Part model, mm, in its own coordinate system. A direction names the side the tool comes from. Give positions to 0.01 mm unless a question says otherwise; leave off trailing zeros. Write each loop counter-clockwise with the first axis right and the second up, starting at its lowest first coordinate (ties: lowest second). Pieces come first, ordered by that corner, then holes. Notation, with made-up numbers: (73.5, 71) - (130.5, 71) arc R24 ccw to (130.5, 93) - close; hole circle Ø5 at (18, 8). An arc over 180 degrees is marked (long way). Answer as a JSON object with one key per item and string values. Group by question number.
```python
from build123d import *


with BuildPart() as part:
    # Sketch1 → Revolve1 (revolve)
    with BuildSketch(Plane.XY):
        with BuildLine():
            Line((-27, 10), (12, 10))
            ThreePointArc((12, 10), (12.707106781, 10.292893219), (13, 11))
            Line((13, 11), (13, 14))
            Line((13, 14), (27, 14))
            Line((27, 14), (27, 17.5))
            Line((27, 17.5), (14, 17.5))
            Line((14, 17.5), (14, 19))
            Line((14, 19), (0, 19))
            Line((0, 19), (0, 21))
            Line((0, 21), (-2, 21))
            Line((-2, 21), (-2, 20.229142798))
            ThreePointArc((-2, 20.229142798), (-2.062403045, 20.049198361), (-2.222815548, 19.946524269))
            Line((-2.222815548, 19.946524269), (-27, 14))
            Line((-27, 14), (-27, 10))
        make_face()
    revolve(axis=Axis((-27, 0, 0), (1, 0, 0)))


solid = part.part
```
1) Mould opens along Z. For faces 4 (the flat face through (13, -6.2, -9.3)), 5 (the cylindrical face through (20.098, 12.932, -5.362)), 6 (the cylindrical face through (-1.01, 20.03, 6.31)), 7 (the flat face through (27, 8, 12)) say: pulls with the +Z half, pulls with the -Z half, needs draft (parallel to the pull), parting line crosses it, or undercut.
2) Drop flat-ended pins along their axis: P1, Ø6, axis at x = -19, z = -13.5, coming from the +Y side; P2, Ø1.5, axis at x = -11, y = -7, coming from the -Z side; P3, Ø6, axis at x = -17.5, z = 4, coming from the -Y side. Give the stop position or say it passes through.
3) Probe line 1 (Z direction, x = 22.5, y = 0); line 2 (X direction, y = -4, z = 13); line 3 (X direction, y = 15.5, z = 13). List the from-to ranges inside material, lowest first.
4) Band-saw the part on C-C (x = -13). List the corners of the cut face in (y, z).
5) Band-saw the part on D-D (x = -21). List the corners of the cut face in (y, z), plus the area to 3 significant figures.
6) Which spindle directions (+Z, -Z, +X, -X, +Y, -Y) get a long thin tool onto all of the face, cutting with end or side? Do faces 1 (the flat face through (-27, -3, 10)), 2 (the flat face through (-2, -11, 17.2)), 3 (the cylindrical face through (20.409, -13.887, -10.648)). Say none if no direction does.
7) Band-saw the part on A-A (z = 0). List the corners of the cut face in (x, y), plus the area to 3 significant figures.
Verdict:
{
 "1": {"face 4": "undercut", "face 5": "undercut", "face 6": "parting line crosses it", "face 7": "needs draft"},
 "2": {"P1": "y = 12.14", "P2": "z = -16.77", "P3": "y = -16.72"},
 "3": {"line 1": "-17.5 to -14, 14 to 17.5", "line 2": "-27 to 13", "line 3": "-2 to 0"},
 "4": {"outline": "circle Ø34.72 at (0, 0); hole circle Ø20 at (0, 0)"},
 "5": {"outline": "circle Ø30.88 at (0, 0); hole circle Ø20 at (0, 0)", "area": "435 mm2"},
 "6": {"face 1": "+Z, -Z, -X, +Y, -Y", "face 2": "-X", "face 3": "+X"},
 "7": {"outline": "(-27, -14) - (-2.22, -19.95) arc R0.29 cw to (-2, -20.23) - (-2, -21) - (0, -21) - (0, -19) - (14, -19) - (14, -17.5) - (27, -17.5) - (27, -14) - (13, -14) - (13, -11) arc R1 ccw to (12, -10) - (-27, -10) - close; (-27, 10) - (12, 10) arc R1 ccw to (13, 11) - (13, 14) - (27, 14) - (27, 17.5) - (14, 17.5) - (14, 19) - (0, 19) - (0, 21) - (-2, 21) - (-2, 20.23) arc R0.29 cw to (-2.22, 19.95) - (-27, 14) - close", "area": "729 mm2"}
}
